Source: CAD feature listing. Evaluate the final solid. Frame: model axes, mm. Face numbers are marked on the shaded views. Give positions to 0.01 mm unless a question says otherwise; leave off trailing zeros. Write each loop counter-clockwise with the first axis right and the second up, starting at its lowest first coordinate (ties: lowest second). Pieces come first, ordered by that corner, then holes. Notation, with made-up numbers: (84.5, 53) -> (112.5, 53) arc R17 cw to (112.5, 66) -> close; hole circle Ø11 at (27, 44.5). An arc over 180 degrees is marked (long way). Answer as a JSON object with one key per item and string values. Group by question number.
Item 1: Section query A-A on y = 0. Return the cut outline in (x, z), plus the area to 3 significant figures.
Item 2: Ray query, probe 1 along X at (y, z) = (-58.5, 5.5); probe 2 along X at (y, z) = (4, 4); probe 3 along Y at (x, z) = (56, 5.5). Return the intervals inside material, ascending. Write a range as from..to.
Item 3: First-contact query: pin 1 Ø1.5 at (x, z) = (9.5, 4) entering from -Y; pin 2 Ø12 at (x, y) = (-39.5, -35.5) entering from +Z. Flat tips, straight axial feed; report the tip coordinate or a pass-through.
Item 4: Pull-direction query (Y, two-part tool) for the marked faces 1, 2 and 3; classes: pulls with the +Y half, pulls with the -Y half, needs draft (parallel to the pull), parting line crosses it, or undercut.
Item 5: Section query B-B on x = 39. Return the cut outline in (y, z), plus the area to 3 significant figures.
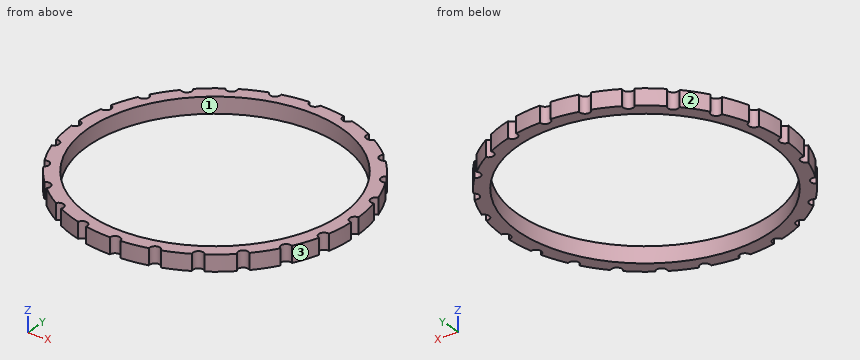
from build123d import *

# Parameters (mm, degrees)
CYLINDER001002001_R              = 2.6
CYLINDER001002001_DEPTH          = 20
CYLINDER001002001001_R           = 2.6
CYLINDER001002001001_DEPTH       = 20
CYLINDER001002001001001_R        = 2.6
CYLINDER001002001001001_DEPTH    = 20
CYLINDER001002001001001001_R     = 2.6
CYLINDER001002001001001001_DEPTH = 26
CYLINDER001002_R                 = 2.6
CYLINDER001002_DEPTH             = 20
CYLINDER001001_R                 = 2.6
CYLINDER001001_DEPTH             = 20
CYLINDER001_R                    = 2.6
CYLINDER001_DEPTH                = 20
CYLINDER002_R                    = 63
CYLINDER002_DEPTH                = 10
CYLINDER_R                       = 70
CYLINDER_DEPTH                   = 8


with BuildPart() as pole2:
    # Cylinder001002001 → Cylinder001002001 (new body)
    with BuildSketch(Plane(origin=(67.55, 18.2, 0), x_dir=(1, 0, 0), z_dir=(0, 0, 1))):
        Circle(CYLINDER001002001_R)
    extrude(amount=CYLINDER001002001_DEPTH)


with BuildPart() as pole003:
    # Cylinder001002001001 → Cylinder001002001001 (new body)
    with BuildSketch(Plane(origin=(60.62, 35, 0), x_dir=(1, 0, 0), z_dir=(0, 0, 1))):
        Circle(CYLINDER001002001001_R)
    extrude(amount=CYLINDER001002001001_DEPTH)


with BuildPart() as pole004:
    # Cylinder001002001001001 → Cylinder001002001001001 (new body)
    with BuildSketch(Plane(origin=(49.49, 49.49, 0), x_dir=(1, 0, 0), z_dir=(0, 0, 1))):
        Circle(CYLINDER001002001001001_R)
    extrude(amount=CYLINDER001002001001001_DEPTH)


with BuildPart() as pole005:
    # Cylinder001002001001001001 → Cylinder001002001001001001 (new body)
    with BuildSketch(Plane(origin=(35, 60.62, 0), x_dir=(1, 0, 0), z_dir=(0, 0, 1))):
        Circle(CYLINDER001002001001001001_R)
    extrude(amount=CYLINDER001002001001001001_DEPTH)


with BuildPart() as cylinder001002:
    # Cylinder001002 → Cylinder001002 (new body)
    with BuildSketch(Plane(origin=(18.2, 67.55, 0), x_dir=(1, 0, 0), z_dir=(0, 0, 1))):
        Circle(CYLINDER001002_R)
    extrude(amount=CYLINDER001002_DEPTH)


with BuildPart() as fusion:
    # Fusion base: copy of pole2
    add(pole2.part)

    # Fusion: union pole003, pole004, pole005, Cylinder001002
    add(pole003.part)
    add(pole004.part)
    add(pole005.part)
    add(cylinder001002.part)


with BuildPart() as part_mirroring001:
    # Part__Mirroring001: instance of Fusion
    add(fusion.part.mirror(Plane(origin=(3e-06, 42.766762, 16), x_dir=(0, -1, 0), z_dir=(1, 0, 0))))


with BuildPart() as part_mirroring001_1:
    # Part__Mirroring001 placement: moved
    add(part_mirroring001.part.moved(Location((0, 0, -2))))


with BuildPart() as cylinder001001:
    # Cylinder001001 → Cylinder001001 (new body)
    with BuildSketch(Plane(origin=(0, 70, 0), x_dir=(1, 0, 0), z_dir=(0, 0, 1))):
        Circle(CYLINDER001001_R)
    extrude(amount=CYLINDER001001_DEPTH)


with BuildPart() as pole1:
    # Cylinder001 → Cylinder001 (new body)
    with BuildSketch(Plane(origin=(70, 0, 0), x_dir=(1, 0, 0), z_dir=(0, 0, 1))):
        Circle(CYLINDER001_R)
    extrude(amount=CYLINDER001_DEPTH)


with BuildPart() as part_mirroring003:
    # Part__Mirroring003: instance of pole1
    add(pole1.part.mirror(Plane(origin=(0, 0, 0), x_dir=(0, -1, 0), z_dir=(1, 0, 0))))


with BuildPart() as part_mirroring003_1:
    # Part__Mirroring003 placement: moved
    add(part_mirroring003.part.moved(Location((0, 0, -3))))


with BuildPart() as part_mirroring:
    # Part__Mirroring: instance of Fusion
    add(fusion.part.mirror(Plane(origin=(42.875, 2e-06, 12.999999), x_dir=(1, 0, 0), z_dir=(0, 1, 0))))


with BuildPart() as part_mirroring_1:
    # Part__Mirroring placement: moved
    add(part_mirroring.part.moved(Location((0, 0, -5))))


with BuildPart() as part_mirroring004:
    # Part__Mirroring004: instance of Cylinder001001
    add(cylinder001001.part.mirror(Plane(origin=(0, 0, 0), x_dir=(1, 0, 0), z_dir=(0, 1, 0))))


with BuildPart() as part_mirroring004_1:
    # Part__Mirroring004 placement: moved
    add(part_mirroring004.part.moved(Location((0, 0, -4))))


with BuildPart() as part_mirroring002:
    # Part__Mirroring002: instance of Part__Mirroring
    add(part_mirroring_1.part.mirror(Plane(origin=(0, 0, 0), x_dir=(0, -1, 0), z_dir=(1, 0, 0))))


with BuildPart() as part_mirroring002_1:
    # Part__Mirroring002 placement: moved
    add(part_mirroring002.part.moved(Location((0, 0, -4))))


with BuildPart() as fusion001:
    # Fusion001 base: copy of Cylinder001002
    add(cylinder001002.part)

    # Fusion001: union pole2, Part__Mirroring001, Cylinder001001, pole005, Part__Mirroring003, Part__Mirroring, Fusion, Part__Mirroring004, pole003, pole1, Part__Mirroring002, pole004
    add(pole2.part)
    add(part_mirroring001_1.part)
    add(cylinder001001.part)
    add(pole005.part)
    add(part_mirroring003_1.part)
    add(part_mirroring_1.part)
    add(fusion.part)
    add(part_mirroring004_1.part)
    add(pole003.part)
    add(pole1.part)
    add(part_mirroring002_1.part)
    add(pole004.part)


with BuildPart() as cylinder002:
    # Cylinder002 → Cylinder002 (new body)
    with BuildSketch(Plane.XY):
        Circle(CYLINDER002_R)
    extrude(amount=CYLINDER002_DEPTH)


with BuildPart() as cut001:
    # Cylinder → Cylinder (new body)
    with BuildSketch(Plane.XY):
        Circle(CYLINDER_R)
    extrude(amount=CYLINDER_DEPTH)

    # Cut: cut Cylinder002
    add(cylinder002.part, mode=Mode.SUBTRACT)

    # Cut001: cut Fusion001
    add(fusion001.part, mode=Mode.SUBTRACT)


solid = cut001.part
Worked answers:
{
 "1": {"outline": "(-67.4, 0) -> (-63, 0) -> (-63, 8) -> (-67.4, 8) -> close; (63, 0) -> (67.4, 0) -> (67.4, 8) -> (63, 8) -> close", "area": "70.4 mm^2"},
 "2": {"probe 1": "-38.44..-36.51, -33.49..-23.38, 23.38..33.49, 36.51..38.44", "probe 2": "-69.89..-62.87, 62.87..69.89", "probe 3": "-42..-28.86, 28.86..42"},
 "3": {"pin 1": "y = -69.45", "pin 2": "through"},
 "4": {"face 1": "undercut", "face 2": "pulls with the +Y half", "face 3": "pulls with the -Y half"},
 "5": {"outline": "(-58.13, 0) -> (-49.48, 0) -> (-49.48, 8) -> (-58.13, 8) -> close; (49.48, 0) -> (58.13, 0) -> (58.13, 8) -> (49.48, 8) -> close", "area": "138 mm^2"}
}
